```python
from build123d import *

# Parameters (mm, degrees)
CROQUIS1_W              = 88.9
CROQUIS1_H              = 25
SALIENTE_EXTRUIR1_DEPTH = 60
CROQUIS2_W              = 88.9
CROQUIS2_H              = 25
CORTAR_EXTRUIR1_DEPTH   = 100


with BuildPart() as part:
    # Croquis1 → Saliente-Extruir1 (new body)
    with BuildSketch(Plane.XY):
        with Locations((44.45, 12.5)):
            Rectangle(CROQUIS1_W, CROQUIS1_H)
    extrude(amount=-SALIENTE_EXTRUIR1_DEPTH)

    # Barrer1: sweep along a curve in space
    with BuildLine() as barrer1_path:
        Line((44.45, 202.5, -590), (44.45, 12.5, -60))
    # Croquis2 → Barrer1 (sweep)
    with BuildSketch(Plane(origin=(0, 0, -60), x_dir=(-1, 0, 0), z_dir=(0, 0, -1))):
        with Locations((-44.45, 12.5)):
            Rectangle(CROQUIS2_W, CROQUIS2_H)
    sweep(path=barrer1_path.line)

    # Croquis3 → Cortar-Extruir1 (cut)
    with BuildSketch(Plane(origin=(0, 25, 0), x_dir=(1, 0, 0), z_dir=(0, 1, 0))):
        Polygon((0, 0), (88.9, 40), (88.9, 0), align=None)
    extrude(amount=-CORTAR_EXTRUIR1_DEPTH, mode=Mode.SUBTRACT)


solid = part.part
```
Can you work these out from the model? Positions are in its coordinate system, mm. A direction names the side the tool comes from. Give positions to 0.01 mm unless a question says otherwise; leave off trailing zeros. Order: outer loops, then holes, each group sorted by start corner. A loop starts at its lowest first (then second) coordinate and runs counter-clockwise, first axis right, second up. Notation, with made-up numbers: (20.5, 38) - (63.5, 38) arc R16 cw to (63.5, 54) - close; hole circle Ø6 at (43.25, -3.5). An arc over 180 degrees is marked (long way). Use a Markdown table: item, result. Add a question column.
Q1. I'm going to push flat-ended pins straight in: pin 1 (18 mm diameter, centred on x = 45, z = -29, fed in from +Y); pin 2 (12 mm diameter, centred on x = 29, z = -147.5, fed in from -Y); pin 3 (5 mm diameter, centred on x = 21.5, z = -198.5, fed in from +Y); pin 4 (12 mm diameter, centred on x = 22, z = -64, fed in from -Y). Where does each tip first touch, or does it pass through?
Q2. If we section it at C-C on y = 128.5: Write out the boundary of the cut face in (x, z), plus the area to 3 significant figures.
Q3. If we section it at A-A on x = 10.5: Write out the boundary of the cut face in (y, z).
Q4. If we section it at B-B on z = -413.5: Write out the boundary of the cut face in (x, y), plus the area to 3 significant figures.
Q5. If we section it at D-D on x = 64.5: Write out the boundary of the cut face in (y, z), plus the area to 3 significant figures.
Q6. On a 3-axis mill with a long thin cutter (end or side, diameter ignored), from which of +Z, -Z, +X, -X, +Y, -Y can I reach the whole of each face in a straight line? I mean faces 1 (the flat face through (43.83, 12.68, -19.72)), 2 (the flat face through (34, 25, -36)). Say none if no direction works.
Q7. Please list where these lines run through material, in increasing order: line 1 along Y through (x, z) = (66.5, -141); line 2 along Y through (x, z) = (5.5, -433).
Answers follow:
| question | item | result |
|---|---|---|
| 1 | pin 1 | stops at y = 25 |
| 1 | pin 2 | stops at y = 29.22 |
| 1 | pin 3 | stops at y = 75.55 |
| 1 | pin 4 | stops at y = 0 |
| 2 | outline | (0, -418.45) - (88.9, -418.45) - (88.9, -348.71) - (0, -348.71) - close |
| 2 | area | 6,200 mm^2 |
| 3 | outline | (0, -60) - (190, -590) - (215, -590) - (25, -60) - (25, -4.72) - (0, -4.72) - close |
| 4 | outline | (0, 126.73) - (88.9, 126.73) - (88.9, 151.73) - (0, 151.73) - close |
| 4 | area | 2,220 mm^2 |
| 5 | outline | (0, -60) - (190, -590) - (215, -590) - (25, -60) - (25, -29.02) - (0, -29.02) - close |
| 5 | area | 14,000 mm^2 |
| 6 | face 1 | +Z, +X, +Y, -Y |
| 6 | face 2 | +Z, +X, -X, +Y |
| 7 | line 1 | y = 29.04 to 54.04 |
| 7 | line 2 | y = 133.72 to 158.72 |
